Autodesk Inventor part; units mm, degrees
ref_plane "YZ Plane" through (0, 0, 0) normal (1, 0, 0) x (0, 1, 0)
ref_plane "XZ Plane" through (0, 0, 0) normal (0, 1, 0) x (-1, 0, 0)
ref_plane "XY Plane" through (0, 0, 0) normal (0, 0, 1) x (1, 0, 0)
sketch "Sketch1" plane through (0, 0, 0) normal (1, 0, 0) x (0, 1, 0)
  line L0 (0, 0) -> (155.1, 0)
  line L1 (155.1, 0) -> (155.1, -10)
  line L2 (0, -20) -> (0, 0)
  line L3 (155.1, -10) -> (101.6, -10)
  line L4 (101.6, -10) -> (101.6, -20)
  line L5 (101.6, -20) -> (0, -20)
  dimension "d3" = 53.5
  dimension "d4" = 155.1
  dimension "d5" = 10
  dimension "d6" = 10
  dimension "d7" = 20
  dimension "d18" = 101.6
extrude "Extrusion1" add sketch "Sketch1" along normal blind 1238.8342
chamfer "Chamfer1" distance 19.812 angle 45 1 edges at (1238.8342, 50.8, -20)
chamfer "Chamfer2" distance 19.812 angle 45 1 edges at (0, 50.8, -20)
properties part number "SkinnySideLength" material "Wood (Birch)"
The listing builds one solid part. Answer for the finished solid, in the listing's coordinates (mm). A direction names the side the tool comes from. Coordinates: 2 decimals unless noted, no trailing zeros. Loops run counter-clockwise (first coordinate to the right, second up) from the corner with the lowest first, then second, coordinate; pieces in that order, holes last. Notation, with made-up numbers: (-3, 68.5) - (43, 68.5) arc R16 cw to (43, 87.5) - close; hole circle Ø10 at (31, 36). An arc over 180 degrees is marked (long way). Use a Markdown table: item, result. Add a question column.
1) For faces 4 (the flat face through (611, 129, -10)), 5 (the flat face through (611, 52, -20)), determine the directions among +Z, -Z, +X, -X, +Y, -Y from which every point of the face is accessible in a straight line to the end or side of a thin tool.
2) The part is cut by section A-A, the plane x = 313. Give the vertices of the cut face in (y, z), and give its area (3 significant figures).
3) The mould has two halves that part along Z. Classify faces 1 (the flat face through (611, 76, 0)), 2 (the flat face through (611, 0, -10)), 3 (the flat face through (1229.067, 59.231, -9.955)): released by +Z, released by -Z, zero draft, split by the parting line, or undercut.
4) The part is cut by section C-C, the plane z = -16.5. Give the vertices of the cut face in (x, y), and give its area (3 significant figures).
5) Find the intervals of material crossed by line 1 (Y direction, x = 669, z = -18.75); line 2 (Z direction, x = 449.5, y = 123.5); line 3 (X direction, y = 120.5, z = -9.75), in increasing order.
6) The part is cut by section B-B, the plane y = 61. Give the vertices of the cut face in (x, z).
7) Given pin 1 (10 mm diameter, centred on y = 92, z = -17, fed in from +X); pin 2 (12 mm diameter, centred on y = 120, z = -10, fed in from -X); pin 3 (2 mm diameter, centred on y = 76, z = -15, fed in from +X), each flat-ended and moving along its own axis, determine where each tip first touches the part or whether it passes through.
Here are the results:
| question | item | result |
|---|---|---|
| 1 | face 4 | -Z, +X, -X, +Y |
| 1 | face 5 | -Z, +X, -X, +Y, -Y |
| 2 | outline | (0, -20) - (101.6, -20) - (101.6, -10) - (155.1, -10) - (155.1, 0) - (0, 0) - close |
| 2 | area | 2,570 mm^2 |
| 3 | face 1 | released by +Z |
| 3 | face 2 | zero draft |
| 3 | face 3 | released by -Z |
| 4 | outline | (16.31, 0) - (1222.52, 0) - (1222.52, 101.6) - (16.31, 101.6) - close |
| 4 | area | 123,000 mm^2 |
| 5 | line 1 | y = 0 to 101.6 |
| 5 | line 2 | z = -10 to 0 |
| 5 | line 3 | x = 9.56 to 1229.27 |
| 6 | outline | (0, -0.19) - (19.81, -20) - (1219.02, -20) - (1238.83, -0.19) - (1238.83, 0) - (0, 0) - close |
| 7 | pin 1 | stops at x = 1227.02 |
| 7 | pin 2 | stops at x = 3.81 |
| 7 | pin 3 | stops at x = 1225.02 |
